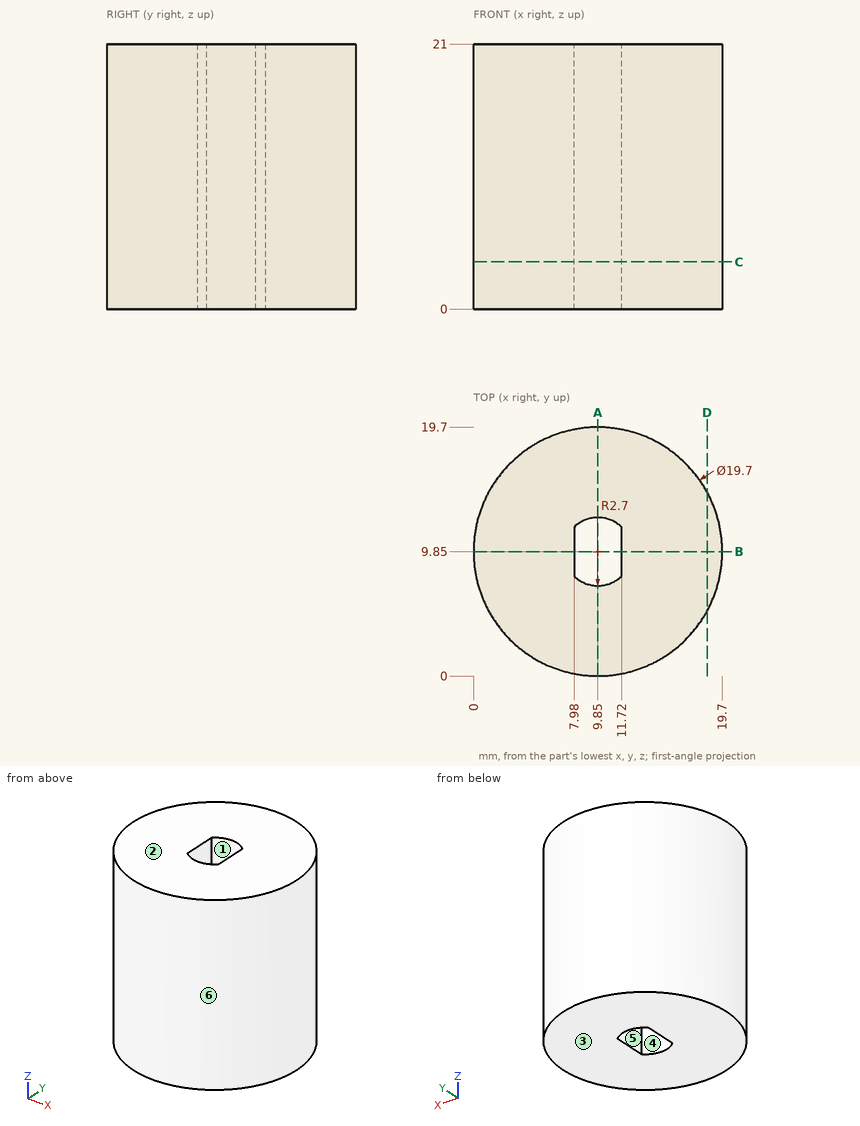
The figure shows three views and two pictorial views of one solid part (mm, origin at its lowest corner). Answer the questions. A direction names the side the tool comes from. Give positions to 0.01 mm unless a question says otherwise; leave off trailing zeros. Loops run counter-clockwise (first coordinate to the right, second up) from the corner with the lowest first, then second, coordinate; pieces in that order, holes last. Notation, with made-up numbers: (28.5, -26) - (33.5, -26) arc R19 cw to (33.5, 4) - close; hole circle Ø6 at (5.5, -10). An arc over 180 degrees is marked (long way). Answer in a Markdown table with one row per item.
(1) Section D-D (x = 18.5) is taken. Give the vertices of the cut face in (y, z), and give its area (3 significant figures).
Results list:
| item | result |
|---|---|
| outline | (5.14, 0) - (14.56, 0) - (14.56, 21) - (5.14, 21) - close |
| area | 198 mm² |
(2) Section C-C (z = 3.75) is taken. Give the vertices of the cut face in (x, y).
Results list:
| item | result |
|---|---|
| outline | circle Ø19.7 at (9.85, 9.85); hole (7.98, 7.9) arc R2.7 ccw to (11.72, 7.9) - (11.72, 11.8) arc R2.7 ccw to (7.98, 11.8) - close |
(3) Flat-ended cylindrical pins translate along their axes: pin 1 Ø2 at (y, z) = (16.5, 18.5) entering from +X; pin 2 Ø5 at (x, z) = (13.5, 7) entering from -Y; pin 3 Ø8 at (y, z) = (17.5, 4.5) entering from -X. Find the tip coordinate at first contact, or state that the pin passes through.
Results list:
| item | result |
|---|---|
| pin 1 | stops at x = 17.92 |
| pin 2 | stops at y = 0.07 |
| pin 3 | stops at x = 0.7 |
(4) Section B-B (y = 9.85) is taken. Give the vertices of the cut face in (x, z).
Results list:
| item | result |
|---|---|
| outline | (0, 0) - (7.98, 0) - (7.98, 21) - (0, 21) - close; (11.72, 0) - (19.7, 0) - (19.7, 21) - (11.72, 21) - close |
(5) Section A-A (x = 9.85) is taken. Give the vertices of the cut face in (y, z).
Results list:
| item | result |
|---|---|
| outline | (0, 0) - (7.15, 0) - (7.15, 21) - (0, 21) - close; (12.55, 0) - (19.7, 0) - (19.7, 21) - (12.55, 21) - close |
(6) For a pull along X with two mould halves and no side action, classify the marked faces 3, 4, 5 and 6 as pulls with the +X half, pulls with the -X half, needs draft (parallel to the pull), parting line crosses it, or undercut.
Results list:
| item | result |
|---|---|
| face 3 | needs draft |
| face 4 | undercut |
| face 5 | undercut |
| face 6 | parting line crosses it |
(7) A tool of negligible diameter and unlimited length cuts with its end or side. For the marked faces 1 and 2, from which of +Z, -Z, +X, -X, +Y, -Y can it reach the whole face along a straight path? Write none if from no direction.
Results list:
| item | result |
|---|---|
| face 1 | +Z, -Z |
| face 2 | +Z, +X, -X, +Y, -Y |
(8) Consider L1, parallel to X at y = 9.75, z = 5; L2, parallel to X at y = 11, z = 6.75; L3, parallel to Y at x = 8.75, z = 7. Determine where each line is inside the solid, lowest interval first. Write a range as [from, to].
Results list:
| item | result |
|---|---|
| L1 | x = [0, 7.98], [11.72, 19.7] |
| L2 | x = [0.07, 7.98], [11.72, 19.63] |
| L3 | y = [0.06, 7.38], [12.32, 19.64] |
